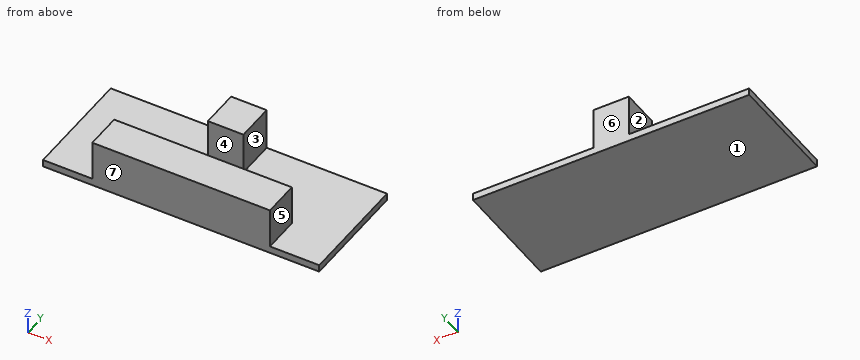
```python
from build123d import *

# Parameters (mm, degrees)
SKETCH1_W           = 62.2
SKETCH1_H           = 25.4
PCB_DEPTH           = 1.6
SKETCH2_W           = 40
SKETCH2_H           = 8.2
SERVO_HEADERS_DEPTH = 9
SKETCH3_W           = 8
SKETCH3_H           = 8.7
V_TERMINAL_DEPTH    = 9.4


with BuildPart() as part:
    # Sketch1 → PCB (new body)
    with BuildSketch(Plane.XY):
        Rectangle(SKETCH1_W, SKETCH1_H)
    extrude(amount=PCB_DEPTH)

    # Sketch2 → Servo_headers (add)
    with BuildSketch(Plane.XY.offset(1.6)):
        with Locations((0, -8.6)):
            Rectangle(SKETCH2_W, SKETCH2_H)
    extrude(amount=SERVO_HEADERS_DEPTH)

    # Sketch3 → V+_terminal (add)
    with BuildSketch(Plane.XY.offset(1.6)):
        with Locations((0, 8.35)):
            Rectangle(SKETCH3_W, SKETCH3_H)
    extrude(amount=V_TERMINAL_DEPTH)


solid = part.part
```
The listing builds one solid part. Answer for the finished solid, in the listing's coordinates (mm). Face numbers are marked on the shaded views. A direction names the side the tool comes from. Give positions to 0.01 mm unless a question says otherwise; leave off trailing zeros. Write each loop counter-clockwise with the first axis right and the second up, starting at its lowest first coordinate (ties: lowest second). Pieces come first, ordered by that corner, then holes. Notation, with made-up numbers: (37, 1.5) -> (59, 1.5) arc R19 cw to (59, 33.5) -> close; hole circle Ø10 at (71.5, 75.5). An arc over 180 degrees is marked (long way). Use one line per item in the form item = value.
1) Section C-C on x = -16.5 is taken. Write down the section's boundary in (y, z).
Result:
outline = (-12.7, 0) -> (12.7, 0) -> (12.7, 1.6) -> (-4.5, 1.6) -> (-4.5, 10.6) -> (-12.7, 10.6) -> close
2) Section A-A on z = 6.25 is taken. Write down the section's boundary in (x, y), plus the area to 3 significant figures.
Result:
outline = (-20, -12.7) -> (20, -12.7) -> (20, -4.5) -> (-20, -4.5) -> close; (-4, 4) -> (4, 4) -> (4, 12.7) -> (-4, 12.7) -> close
area = 398 mm²
3) Section D-D on y = -8 is taken. Write down the section's boundary in (x, z).
Result:
outline = (-31.1, 0) -> (31.1, 0) -> (31.1, 1.6) -> (20, 1.6) -> (20, 10.6) -> (-20, 10.6) -> (-20, 1.6) -> (-31.1, 1.6) -> close
4) Section B-B on y = 9.5 is taken. Write down the section's boundary in (x, z).
Result:
outline = (-31.1, 0) -> (31.1, 0) -> (31.1, 1.6) -> (4, 1.6) -> (4, 11) -> (-4, 11) -> (-4, 1.6) -> (-31.1, 1.6) -> close
5) A tool of negligible diameter and unlimited length cuts with its end or side. For the marked faces 1, 2 and 3, from which of +Z, -Z, +X, -X, +Y, -Y can it reach the whole face along a straight path? Write none if from no direction.
Result:
face_1 = -Z, +X, -X, +Y, -Y
face_2 = +Z, -X, +Y
face_3 = +Z, +X, +Y
6) For a pull along Y with two mould halves and no side action, classify the marked faces 4, 5, 6 and 7 as +Y half, -Y half, draft (parallel to the pull), parting line (faces both ways), or undercut.
Result:
face_4 = undercut
face_5 = draft
face_6 = +Y half
face_7 = -Y half
7) Straight lines are drawn through the part: probe 1 along Y at (x, z) = (-2.5, 2.5); probe 2 along Z at (x, y) = (5, 3.25); probe 3 along Z at (x, y) = (16, -7.5). For each, find the intervals that lie inside material, in ascending order.
Result:
probe_1 = -12.7 to -4.5, 4 to 12.7
probe_2 = 0 to 1.6
probe_3 = 0 to 10.6
8) Each of these flat-tipped pins is pushed along its axis until it touches: P1, Ø4.5, axis at y = 6, z = 4.5, coming from the -X side; P2, Ø5, axis at x = -21, y = 3, coming from the +Z side; P3, Ø4, axis at y = -7, z = 4.5, coming from the +X side. Where does it stop, or does it pass through?
Result:
P1 = -4
P2 = 1.6
P3 = 20
